Check sheet for the modelled part. Datum: model origin and axes. Units: mm. Round coordinates to 2 decimals unless told otherwise and drop trailing zeros. Write each loop counter-clockwise with the first axis right and the second up, starting at its lowest first coordinate (ties: lowest second). Pieces come first, ordered by that corner, then holes. Notation, with made-up numbers: (-12, -27.5) -> (24, -27.5) arc R13 ccw to (24, -16.5) -> close; hole circle Ø2 at (28.5, 77). An arc over 180 degrees is marked (long way). One line per item, written item: value.
from build123d import *

# Parameters (mm, degrees)
F0_W     = 12.7
F0_H     = 63.5
F1_DEPTH = 6.35
F0_W_2   = 50.8
F0_H_2   = 228.6
F2_DEPTH = 25.4
F4_D     = 7.62


with BuildPart() as f1:
    # F0 (on Top) → F1 (new body)
    with BuildSketch(Plane.XY):
        with Locations((-38.724346, 73.146781)):
            Rectangle(F0_W, F0_H)
    extrude(amount=F1_DEPTH)

    # F0 (on Top) → F2 (join)
    with BuildSketch(Plane.XY):
        with Locations((-38.724346, 9.646781)):
            Rectangle(F0_W_2, F0_H_2)
        with Locations((-38.724346, 73.146781)):
            Rectangle(F0_W, F0_H, mode=Mode.SUBTRACT)
    extrude(amount=F2_DEPTH)

    # F4 (through all)
    with Locations(Plane(origin=(-64.124346, 0, 0), x_dir=(0, -1, 0), z_dir=(-1, 0, 0))):
        with Locations((92.579484, 14.321566)):
            Hole(F4_D / 2)


solid = f1.part
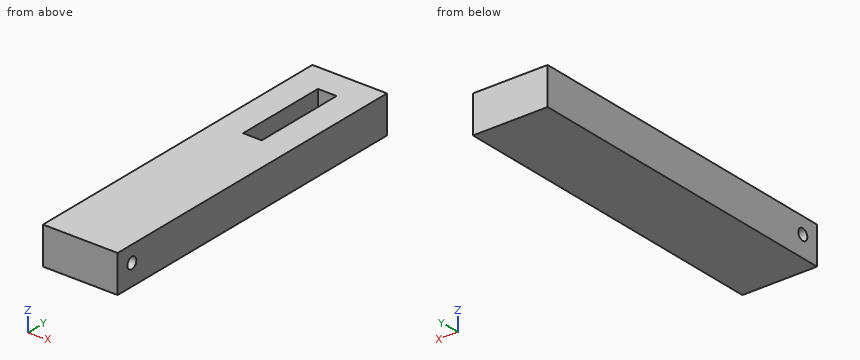
Item 1: Depth check by flat-ended pin: P1, Ø6.5, axis at x = -40.5, y = 58.5, coming from the +Z side. Enter the tip coordinate at first touch or a pass-through.
Answer:
P1: stops at z = 6.35
Item 2: Thickness scan on line 1 (X direction, y = 50, z = 14.75); line 2 (Y direction, x = -22.5, z = 12.25); line 3 (Y direction, x = -53, z = 11.25). Record the ranges inside material, lowest first.
Answer:
line 1: x = -64.12 to -45.07, -32.37 to -13.32
line 2: y = -104.65 to -95.78, -89.38 to 123.95
line 3: y = -104.65 to -94.83, -90.33 to 123.95
Item 3: Sectioned sample at B-B on y = 97.5. Enter the section's corners in (x, z), and give its area (3 significant figures).
Answer:
outline: (-64.12, 0) -> (-13.32, 0) -> (-13.32, 25.4) -> (-32.37, 25.4) -> (-32.37, 6.35) -> (-45.07, 6.35) -> (-45.07, 25.4) -> (-64.12, 25.4) -> close
area: 1,050 mm^2
Item 4: Sectioned sample at A-A on z = 22.5. Enter the section's corners in (x, y), and give its area (3 significant figures).
Answer:
outline: (-64.12, -104.65) -> (-13.32, -104.65) -> (-13.32, 123.95) -> (-64.12, 123.95) -> close; hole (-45.07, 41.4) -> (-32.37, 41.4) -> (-32.37, 104.9) -> (-45.07, 104.9) -> close
area: 10,800 mm^2
